Input: part model. Units: mm. Frame: model coordinates. Face numbers are marked on the shaded views. Round coordinates to 2 decimals unless told otherwise and drop trailing zeros. Order: outer loops, then holes, each group sorted by start corner. A loop starts at its lowest first (then second) coordinate and runs counter-clockwise, first axis right, second up.
Item 1: Line query: L1, parallel to X at y = 2.4, z = 0; L2, parallel to X at y = 0.3, z = 0; L3, parallel to X at y = 2.3, z = 10. Output: solid intervals per line, ascending.
Item 2: First-contact query: pin 1 (1 mm diameter, centred on y = 2, z = 0, fed in from -X); pin 2 (1.5 mm diameter, centred on y = -0.5, z = -5.5, fed in from +X); pin 3 (17 mm diameter, centred on x = 0, z = 0, fed in from -Y); pin 4 (1.5 mm diameter, centred on x = -11.5, y = 0, fed in from -Z). Flat tips, straight axial feed; report the tip coordinate or a pass-through.
Item 3: Cut plane C-C on y = 1.4. Output: boundary loops of the cut face in (x, z).
Item 4: Mould query, pull axis Z, two halves, no side actions, for the marked faces 1, 2 and 3. Classes: released by +Z, released by -Z, zero draft, split by the parting line, or undercut.
Item 5: Cut plane B-B on z = 0. Output: boundary loops of the cut face in (x, y), then the cut area to 3 significant figures.
Item 6: Cut plane A-A on x = 0. Output: boundary loops of the cut face in (y, z).
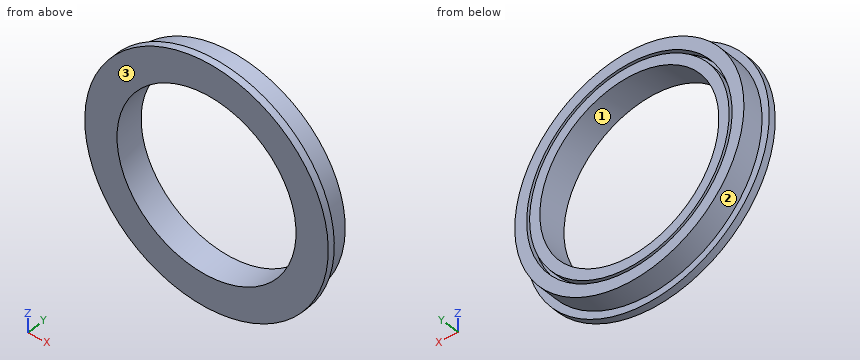
```python
from build123d import *

# Parameters (mm, degrees)
SKETCH_1_W          = 3.5
SKETCH_1_H          = 3
EXTRUDE_START       = 1
SKETCH_2_R          = 17
SKETCH_2_R_2        = 12.5
EXTRUDE_1_DEPTH     = 1
SKETCH_3_R          = 14.340356903
SKETCH_3_R_2        = 13.93231215
CUT_EXTRUDE_1_DEPTH = 1


with BuildPart() as part:
    # 草图1 → 旋转1 (revolve)
    with BuildSketch(Plane.XY, mode=Mode.PRIVATE) as revolve_1_sk:
        with Locations((14.25, 1.5)):
            Rectangle(SKETCH_1_W, SKETCH_1_H)
    revolve(revolve_1_sk.sketch.rotate(Axis((0, 0, 0), (0, 1, 0)), 90), axis=Axis((0, 0, 0), (0, 1, 0)))

    # 草图2 → 凸台-拉伸1 (add)
    with BuildSketch(Plane.XZ.offset(EXTRUDE_START)):
        with Locations(Location((0, 0, 0), (0, 0, 270))):
            Circle(SKETCH_2_R)
        with Locations(Location((0, 0, 0), (0, 0, 270))):
            Circle(SKETCH_2_R_2, mode=Mode.SUBTRACT)
    extrude(amount=-EXTRUDE_1_DEPTH)

    # 草图3 → 切除-拉伸1 (cut)
    with BuildSketch(Plane(origin=(0, 3, 0), x_dir=(1, 0, 0), z_dir=(0, 1, 0))):
        with Locations(Location((0, 0, 0), (0, 0, 270))):
            Circle(SKETCH_3_R)
        with Locations(Location((0, 0, 0), (0, 0, 270))):
            Circle(SKETCH_3_R_2, mode=Mode.SUBTRACT)
    extrude(amount=-CUT_EXTRUDE_1_DEPTH, mode=Mode.SUBTRACT)


solid = part.part
```
From the geometry:
1. L1: x = -16 to -14.34, -13.93 to -12.5, 12.5 to 13.93, 14.34 to 16
1. L2: x = -16 to -12.5, 12.5 to 16
1. L3: x = -12.49 to -10.28, -9.7 to -7.5, 7.5 to 9.7, 10.28 to 12.49
2. pin 1: stops at x = -16
2. pin 2: stops at x = 16.32
2. pin 3: passes through
2. pin 4: stops at z = -13.17
3. outline: circle Ø32 at (0, 0); hole circle Ø25 at (0, 0)
4. face 1: undercut
4. face 2: split by the parting line
4. face 3: zero draft
5. outline: (-17, -1) - (-12.5, -1) - (-12.5, 3) - (-13.93, 3) - (-13.93, 2) - (-14.34, 2) - (-14.34, 3) - (-16, 3) - (-16, 0) - (-17, 0) - close; (12.5, -1) - (17, -1) - (17, 0) - (16, 0) - (16, 3) - (14.34, 3) - (14.34, 2) - (13.93, 2) - (13.93, 3) - (12.5, 3) - close
5. area: 29.2 mm2
6. outline: (-1, -17) - (0, -17) - (0, -16) - (3, -16) - (3, -14.34) - (2, -14.34) - (2, -13.93) - (3, -13.93) - (3, -12.5) - (-1, -12.5) - close; (-1, 12.5) - (3, 12.5) - (3, 13.93) - (2, 13.93) - (2, 14.34) - (3, 14.34) - (3, 16) - (0, 16) - (0, 17) - (-1, 17) - close
